Geometry: final body of the model. Coordinates: model frame, mm. A direction names the side the tool comes from. Round coordinates to 2 decimals unless told otherwise and drop trailing zeros. Write each loop counter-clockwise with the first axis right and the second up, starting at its lowest first coordinate (ties: lowest second). Pieces come first, ordered by that corner, then holes. Notation, with made-up numbers: M -26,57.25 L -16,57.25 A20 cw -16,78.25 Z; hole C 23,10 d10. An arc over 180 degrees is marked long. Use one line per item in the form item = value. Start each with the question number.
from build123d import *

# Parameters (mm, degrees)
SKETCH001_R     = 4
POCKET_DEPTH    = 23.001
CHAMFER_SIZE    = 3.5
CHAMFER001_SIZE = 4
SKETCH002_R     = 2.5
POCKET001_DEPTH = 100.001


with BuildPart() as part:
    # Sketch → Revolution (revolve)
    with BuildSketch(Plane.XZ):
        Polygon((0, 15), (0, 17.5), (11, 17.5), (11, 26), (17, 26), (17, 50), (24, 50), (24, 37), (30, 37), (30, 15), align=None)
    revolve(axis=Axis((0, 0, 0), (1, 0, 0)))

    # Sketch001 → Pocket (cut, through all)
    with BuildSketch(Plane(origin=(7, 0, 0), x_dir=(0, 0, -1), z_dir=(-1, 0, 0))):
        with Locations((0, 41.75)):
            Circle(SKETCH001_R)
        with Locations((35.937446, -21.25)):
            Circle(SKETCH001_R)
        with Locations((-35.937446, -21.25)):
            Circle(SKETCH001_R)
    extrude(amount=-POCKET_DEPTH, mode=Mode.SUBTRACT)

    # Chamfer
    chamfer_edges = [part.edges().sort_by_distance(p)[0] for p in [
        (17, -41.75, 4),
        (17, 21.25, 39.937446),
        (17, 21.25, -31.937446),
    ]]
    chamfer(chamfer_edges, length=CHAMFER_SIZE)

    # Chamfer001
    chamfer001_edges = [part.edges().sort_by_distance(p)[0] for p in [
        (30, 0, -15),
    ]]
    chamfer(chamfer001_edges, length=CHAMFER001_SIZE)

    # Sketch002 (on DatumPlane) → Pocket001 (cut, through all)
    with BuildSketch(Plane.XY.offset(50)):
        with Locations((14, 0)):
            Circle(SKETCH002_R)
    extrude(amount=-POCKET001_DEPTH, mode=Mode.SUBTRACT)


solid = part.part
1. Ray query, probe 1 along Y at (x, z) = (20.5, 0); probe 2 along Y at (x, z) = (16.5, 0); probe 3 along Z at (x, y) = (9, 0). Return the intervals inside material, ascending.
2. Pull-direction query (Z, two-part tool) for faces 4 (the face through (26.2, 9.2, -12.1)), 5 (the face through (5.577, 10.648, -13.887)), 6 (the face through (30, -17, -9)); classes: released by +Z, released by -Z, zero draft, split by the parting line, or undercut.
3. Set-up query: faces 1 (the face through (22.23, 20.05, 32.12)), 2 (the face through (11, 17, -5)), 3 (the face through (24, 37, 7)). Return all of +Z, -Z, +X, -X, +Y, -Y with unobstructed straight access to the full face (end or side cutting, diameter ignored); none if empty.
4. Section query C-C (x = 13). Return loops of the section in (y, z).
5. Section query D-D (y = 21.25). Return loops of the section in (x, z).
6. Contact query for flat-ended pins moving along their axis: pin 1 (6 mm diameter, centred on x = 3, z = 21, fed in from -Y); pin 2 (9 mm diameter, centred on y = -41.75, z = 0, fed in from -X); pin 3 (5 mm diameter, centred on x = 18.5, z = -34.5, fed in from +Y); pin 4 (12 mm diameter, centred on x = 13.5, z = 30, fed in from +Y). Output: stop coordinate, or through.
7. Section query A-A (z = 0). Return loops of the section in (x, y), then the cut area to 3 significant figures.
8. Section query B-B (y = 0). Give the number of separate pieces and of enclosed holes in the cut face, then the cut area to 3 significant figures.
Checks:
q1.probe_1 = -50 to -45.75, -37.75 to -15, 15 to 50
q1.probe_2 = -26 to -15, 15 to 26
q1.probe_3 = -17.5 to -15, 15 to 17.5
q2.face_4 = undercut
q2.face_5 = split by the parting line
q2.face_6 = zero draft
q3.face_1 = +X, -X
q3.face_2 = -X
q3.face_3 = +X
q4.outline = M -2.29,-25.9 L -2.29,-14.82 A15 cw -2.29,14.82 L -2.29,25.9 A26 ccw Z; M 2.29,-25.9 A26 ccw 2.29,25.9 L 2.29,14.82 A15 cw 2.29,-14.82 Z
q5.outline = M 11,-14.98 L 17,-14.98 L 17,-28.44 L 20.5,-31.94 L 24,-31.94 L 24,-30.29 L 30,-30.29 L 30,30.29 L 24,30.29 L 24,31.94 L 20.5,31.94 L 17,28.44 L 17,14.98 L 11,14.98 Z; M 17,-45.26 L 24,-45.26 L 24,-39.94 L 20.5,-39.94 L 17,-43.44 Z; M 17,43.44 L 20.5,39.94 L 24,39.94 L 24,45.26 L 17,45.26 Z
q6.pin_1 = through
q6.pin_2 = 20
q6.pin_3 = 38.42
q6.pin_4 = 43.23
q7.outline = M 0,-17.5 L 11,-17.5 L 11,-26 L 17,-26 L 17,-34.25 L 20.5,-37.75 L 24,-37.75 L 24,-37 L 30,-37 L 30,-19 L 26,-15 L 0,-15 Z; M 0,15 L 26,15 L 30,19 L 30,37 L 24,37 L 24,50 L 17,50 L 17,26 L 11,26 L 11,17.5 L 0,17.5 Z; M 17,-50 L 24,-50 L 24,-45.75 L 20.5,-45.75 L 17,-49.25 Z
q7.area = 857 mm^2
q8.separate_pieces = 4
q8.enclosed_holes = 0
q8.area = 815 mm^2
